Geometry check sheet. Reference: the model listing, model coordinates, mm. Round coordinates to 2 decimals unless told otherwise and drop trailing zeros. Loops run counter-clockwise (first coordinate to the right, second up) from the corner with the lowest first, then second, coordinate; pieces in that order, holes last. Notation, with made-up numbers: (-24.5, 32) - (31.5, 32) arc R13 cw to (31.5, 53) - close; hole circle Ø3 at (-20.75, 16.25). An arc over 180 degrees is marked (long way). Answer in a Markdown table with one row per item. Add a question column.
Autodesk Inventor part; units mm, degrees
ref_plane "YZ Plane" through (0, 0, 0) normal (1, 0, 0) x (0, 1, 0)
ref_plane "XZ Plane" through (0, 0, 0) normal (0, 1, 0) x (-1, 0, 0)
ref_plane "XY Plane" through (0, 0, 0) normal (0, 0, 1) x (1, 0, 0)
ref_plane "Work Plane1" through (0, 0, 0) normal (0, 0, 1) x (1, 0, 0)
sketch "Sketch1" plane through (0, 0, 0) normal (0, 0, 1) x (1, 0, 0)
  line L0 (-28.1, 210.2) -> (-28.1, 202.1) construction
  line L1 (-28.1, 202.1) -> (-23.1, 202.1) construction
  line L2 (-23.1, 199.1) -> (-23.1, 202.1) construction
  line L3 (-23.1, 199.1) -> (-123.1, 199.1) construction
  line L4 (-123.1, 199.1) -> (-123.1, 210.2) construction
  line L5 (-28.1, 210.2) -> (-123.1, 210.2) construction
  line L6 (-23.1, -199.1) -> (-23.1, -210.2) construction
  line L7 (-23.1, -210.2) -> (-123.1, -210.2) construction
  line L8 (-123.1, -199.1) -> (-123.1, -210.2) construction
  line L9 (-23.1, -199.1) -> (-123.1, -199.1) construction
  line L10 (23, -210.2) -> (-23, -210.2) construction
  line L11 (-23, -210.2) -> (-23, -202.2) construction
  line L12 (23, -202.2) -> (-23, -202.2) construction
  line L13 (23, -210.2) -> (23, -202.2) construction
  line L14 (28, 202.2) -> (-28, 202.2) construction
  line L15 (-28, 202.2) -> (-28, 210.2) construction
  line L16 (28, 210.2) -> (-28, 210.2) construction
  line L17 (28, 202.2) -> (28, 210.2) construction
  line L18 (7.95, 199) -> (7.95, -199) construction
  line L19 (7.95, -199) -> (-7.95, -199) construction
  line L20 (-7.95, -199) -> (-7.95, 199) construction
  line L21 (-7.95, 199) -> (7.95, 199) construction
  line L22 (-11.95, 199) -> (-11.95, -199) construction
  line L23 (-11.95, -199) -> (-19.95, -199) construction
  line L24 (-19.95, -199) -> (-19.95, 199) construction
  line L25 (-19.95, 199) -> (-11.95, 199) construction
  line L26 (11.95, -199) -> (11.95, 199) construction
  line L27 (11.95, 199) -> (19.95, 199) construction
  line L28 (19.95, 199) -> (19.95, -199) construction
  line L29 (19.95, -199) -> (11.95, -199) construction
  line L30 (-123.1, 210.2) -> (19.95, 210.2)
  line L31 (19.95, 210.2) -> (19.95, 110.2)
  line L32 (19.95, 110.2) -> (-123.1, 110.2)
  line L33 (-123.1, 110.2) -> (-123.1, 210.2)
  circle A0 centre (-9.95, 115.2) radius 2.15
  circle A1 centre (9.95, 115.2) radius 2.15
  circle A2 centre (9.95, 194) radius 2.15
  circle A3 centre (-9.95, 194) radius 2.15
  line L34 (-11.95, 155.8556) -> (-7.95, 155.8556) construction
  line L35 (7.95, 155.8556) -> (11.95, 155.8556) construction
  line L36 (-9.95, 155.8556) -> (-9.95, 110.2) construction
  line L37 (9.95, 155.8556) -> (9.95, 110.2) construction
  line L38 (-89.6001, 199.1) -> (-89.6001, 210.2) construction
  line L39 (-89.6001, 204.65) -> (-123.1, 204.65) construction
  circle A4 centre (-103.1, 204.65) radius 2.65
  circle A5 centre (-83.1, 204.65) radius 2.65
  circle A6 centre (-63.1, 204.65) radius 2.65
  circle A7 centre (-43.1, 204.65) radius 2.65
  point P0 (0, 0)
extrude "Extrusion1" add sketch "Sketch1" along normal blind 10
sketch "Sketch2" plane through (0, 0, 0) normal (0, 0, -1) x (-1, 0, 0)
  circle A0 centre (83.1, 186.5) radius 2.65 construction
  circle A1 centre (98.1, 186.5) radius 2.65 construction
  circle A2 centre (113.1, 186.5) radius 2.65 construction
  circle A3 centre (83.1, 186.5) radius 2.5
  circle A4 centre (98.1, 186.5) radius 2.5
  circle A5 centre (113.1, 186.5) radius 2.5
  point P0 (0, 0)
  dimension "d20" = 5
  dimension "d21" = 5
  dimension "d22" = 5
extrude "Extrusion2" cut sketch "Sketch2" against normal through all
sketch "Sketch3" plane through (0, 0, 10) normal (0, 0, 1) x (1, 0, 0)
  circle A0 centre (-115.6, 141.5) radius 2.65 construction
  circle A1 centre (-115.6, 156.5) radius 2.65 construction
  circle A2 centre (-115.6, 126.5) radius 2.65 construction
  circle A3 centre (-115.6, 171.5) radius 2.65 construction
  arc A4 (-111.2, 191.1249) -> (-111.2, 181.8751) centre (-113.1, 186.5) ccw construction
  line L0 (-111.2, 264.8) -> (-111.2, 191.1249) construction
  line L1 (-111.2, 264.8) -> (-223.2, 264.8) construction
  line L2 (-223.2, 105.1) -> (-223.2, 264.8) construction
  line L3 (-223.2, 105.1) -> (-111.2, 105.1) construction
  line L4 (-111.2, 181.8751) -> (-111.2, 105.1) construction
  circle A5 centre (-115.6, 171.5) radius 2.5
  circle A6 centre (-115.6, 156.5) radius 2.5
  circle A7 centre (-115.6, 141.5) radius 2.5
  circle A8 centre (-115.6, 126.5) radius 2.5
  point P0 (0, 0)
  dimension "d25" = 5
  dimension "d28" = 15
extrude "Extrusion3" cut sketch "Sketch3" against normal through all
equation "\"d2\" = d1"
equation "\"d3\" = d1"
equation "\"d4\" = d1"
equation "\"d6\" = d5"
equation "\"d7\" = d5"
equation "\"d8\" = d5"
properties part number "backboard"
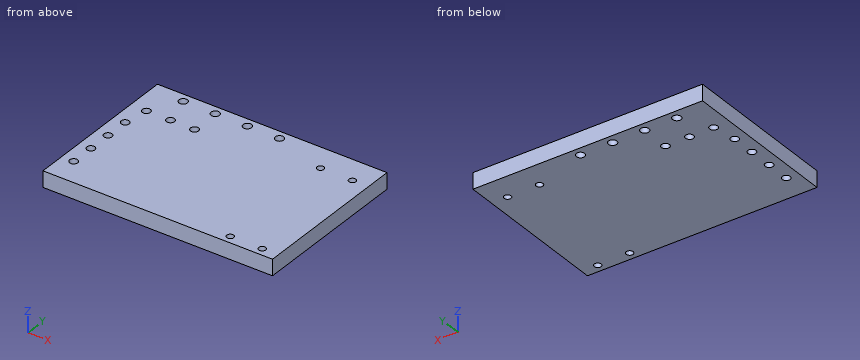
Q1. Scan lines: line 1 (X direction, y = 186.5, z = 6.5); line 2 (Y direction, x = -83.1, z = 5); line 3 (X direction, y = 204.65, z = 7.5). Record each from-to range of solid material in increasing order. Write a range as from..to.
Q2. Cross-section at C-C, the plane y = 126.5. Enter the section's corners in (x, z).
Q3. Depth check by flat-ended pin: P1, Ø4, axis at x = -9.95, y = 115.2, coming from the -Z side. Enter the tip coordinate at first touch or a pass-through.
Q4. Cross-section at A-A, the plane x = -83.1. Enter the section's corners in (y, z), plus the area to 3 significant figures.
Q5. Cross-section at B-B, the plane z = 2.5. State how many separate pieces and enclosed holes the cut face has, plus the area to 3 significant figures.
Q6. Cross-section at D-D, the plane x = -63.1. Enter the section's corners in (y, z), plus the area to 3 significant figures.
Check sheet entries:
| question | item | result |
|---|---|---|
| 1 | line 1 | -123.1..-115.6, -110.6..-100.6, -95.6..-85.6, -80.6..19.95 |
| 1 | line 2 | 110.2..184, 189..202, 207.3..210.2 |
| 1 | line 3 | -123.1..-105.75, -100.45..-85.75, -80.45..-65.75, -60.45..-45.75, -40.45..19.95 |
| 2 | outline | (-123.1, 0) - (-118.1, 0) - (-118.1, 10) - (-123.1, 10) - close; (-113.1, 0) - (19.95, 0) - (19.95, 10) - (-113.1, 10) - close |
| 3 | P1 | through |
| 4 | outline | (110.2, 0) - (184, 0) - (184, 10) - (110.2, 10) - close; (189, 0) - (202, 0) - (202, 10) - (189, 10) - close; (207.3, 0) - (210.2, 0) - (210.2, 10) - (207.3, 10) - close |
| 4 | area | 897 mm² |
| 5 | separate pieces | 1 |
| 5 | enclosed holes | 15 |
| 5 | area | 14,000 mm² |
| 6 | outline | (110.2, 0) - (202, 0) - (202, 10) - (110.2, 10) - close; (207.3, 0) - (210.2, 0) - (210.2, 10) - (207.3, 10) - close |
| 6 | area | 947 mm² |
